Verification items for the finished model (mm, model axes). A direction names the side the tool comes from. Round coordinates to 2 decimals unless told otherwise and drop trailing zeros. Loops run counter-clockwise (first coordinate to the right, second up) from the corner with the lowest first, then second, coordinate; pieces in that order, holes last. Notation, with made-up numbers: (84, -32.75) - (138, -32.75) arc R20 cw to (138, -6.75) - close; hole circle Ø3 at (29.25, -35). An arc over 180 degrees is marked (long way). Use CSV: the item, a comma, the result in double quotes.
```python
from build123d import *

# Parameters (mm, degrees)
F0_W          = 105.625689
F0_H          = 88.043314
F0_R          = 1.5
F1_DEPTH      = 35
F0_W_2        = 44.878527
F2_DEPTH      = 26
F3_SIZE       = 5
F4_W          = 102.581762
F4_H          = 82.043314
F4_W_2        = 41.922454
F5_DEPTH      = 25
F6_R          = 5
F7_W          = 50
F7_H          = 14
F8_DEPTH      = 3
F9_DEPTH      = 25
F9_DEPTH_BACK = 3
F10_W         = 88.043314
F10_H         = 21
F11_DEPTH     = 25


with BuildPart() as f1:
    # F0 (on Top) → F1 (new body)
    with BuildSketch(Plane.XY):
        with Locations((-22.055275, 0)):
            Rectangle(F0_W, F0_H)
        with Locations((-20, -35.20183)):
            Circle(F0_R, mode=Mode.SUBTRACT)
        with Locations((0, -35.20183)):
            Circle(F0_R, mode=Mode.SUBTRACT)
        with Locations((20, -35.20183)):
            Circle(F0_R, mode=Mode.SUBTRACT)
        with Locations((-20, 35.20183)):
            Circle(F0_R, mode=Mode.SUBTRACT)
        with Locations((0, 35.20183)):
            Circle(F0_R, mode=Mode.SUBTRACT)
        with Locations((20, 35.20183)):
            Circle(F0_R, mode=Mode.SUBTRACT)
        with Locations((-20, 35.20183)):
            Circle(F0_R)
        with Locations((0, 35.20183)):
            Circle(F0_R)
        with Locations((20, 35.20183)):
            Circle(F0_R)
        with Locations((20, -35.20183)):
            Circle(F0_R)
        with Locations((0, -35.20183)):
            Circle(F0_R)
        with Locations((-20, -35.20183)):
            Circle(F0_R)
    extrude(amount=F1_DEPTH)

    # F0 (on Top) → F2 (join)
    with BuildSketch(Plane.XY):
        with Locations((53.196832, 0)):
            Rectangle(F0_W_2, F0_H)
    extrude(amount=F2_DEPTH)

    # F3
    f3_edges = [f1.edges().sort_by_distance(p)[0] for p in [
        (30.757569, 0, 35),
    ]]
    chamfer(f3_edges, length=F3_SIZE)

    # F4 (on Top) → F5 (cut)
    with BuildSketch(Plane.XY):
        with Locations((-20.577239, 0)):
            Rectangle(F4_W, F4_H)
        with Locations((51.674869, 0)):
            Rectangle(F4_W_2, F4_H)
    extrude(amount=F5_DEPTH, mode=Mode.SUBTRACT)

    # F6
    f6_edges = [f1.edges().sort_by_distance(p)[0] for p in [
        (53.196833, -44.021657, 26),
        (75.636096, 0, 26),
        (53.196833, 44.021657, 26),
    ]]
    fillet(f6_edges, radius=F6_R)

    # F7 (on face) → F8 (cut)
    with BuildSketch(Plane(origin=(-74.86812, 0, 0), x_dir=(0, -1, 0), z_dir=(-1, 0, 0))):
        with Locations((-5.428568, 10)):
            Rectangle(F7_W, F7_H)
    extrude(amount=-F8_DEPTH, mode=Mode.SUBTRACT)

    # F0 (on Top) → F9 (join, two sides)
    with BuildSketch(Plane.XY) as f9_sk:
        with Locations((-20, -35.20183)):
            Circle(F0_R)
        with Locations((0, -35.20183)):
            Circle(F0_R)
        with Locations((20, -35.20183)):
            Circle(F0_R)
        with Locations((-20, 35.20183)):
            Circle(F0_R)
        with Locations((20, 35.20183)):
            Circle(F0_R)
        with Locations((0, 35.20183)):
            Circle(F0_R)
    extrude(amount=F9_DEPTH)
    extrude(f9_sk.sketch, amount=-F9_DEPTH_BACK)

    # F10 (on face) → F11 (cut)
    with BuildSketch(Plane.YZ.offset(75.636096)):
        with Locations((0, 10.5)):
            Rectangle(F10_W, F10_H)
    extrude(amount=-F11_DEPTH, mode=Mode.SUBTRACT)


solid = f1.part
```
1) Gauge pin test, flat ends, axial feed: pin 1 Ø1.5 at (x, y) = (-5, 27.5) entering from -Z; pin 2 Ø20 at (y, z) = (-3.5, 7.5) entering from +X; pin 3 Ø3.5 at (x, y) = (-73, 12.5) entering from -Z. Record the tip position at first contact, or that the pin passes through.
Returned:
pin 1,"stops at z = 25"
pin 2,"stops at x = -71.87"
pin 3,"stops at z = 0"
2) Cross-section at D-D, the plane y = -32. Record the cut outline in (x, z), then the cut area to 3 significant figures.
Returned:
outline,"(-74.87, 0) - (-71.87, 0) - (-71.87, 25) - (72.64, 25) - (72.64, 21) - (75.64, 21) arc R5 ccw to (70.64, 26) - (30.76, 26) - (30.76, 30) - (25.76, 35) - (-74.87, 35) - close"
area,"1,170 mm²"
3) Mould release check, pull along Y, two halves, no side actions. Record for faces 5 (the face through (53.51, 42.52, 24.57)), 6 (the face through (-73, 6, 17)), 7 (the face through (53.511, -42.596, 24.496)), 8 (the face through (0, 35, -3)): +Y half, -Y half, draft (parallel to the pull), parting line (faces both ways), or undercut.
Returned:
face 5,"+Y half"
face 6,"undercut"
face 7,"-Y half"
face 8,"draft"
4) Cross-section at B-B, the plane z = 13. Record the cut outline in (x, y).
Returned:
outline,"(-74.87, -44.02) - (50.64, -44.02) - (50.64, -41.02) - (-71.87, -41.02) - (-71.87, -19.57) - (-74.87, -19.57) - close; (-74.87, 30.43) - (-71.87, 30.43) - (-71.87, 41.02) - (50.64, 41.02) - (50.64, 44.02) - (-74.87, 44.02) - close; circle Ø3 at (-20, -35.2); circle Ø3 at (-20, 35.2); circle Ø3 at (0, -35.2); circle Ø3 at (0, 35.2); circle Ø3 at (20, -35.2); circle Ø3 at (20, 35.2)"
5) Access from +Z, -Z, +X, -X, +Y, -Y to the whole of each face (thin tool, end or side, straight path). Record for faces 1 (the face through (50.636, 43, 11)), 2 (the face through (-20, 35, -3)), 3 (the face through (50, 1, 26)), 4 (the face through (-71.868, -1, 18)).
Returned:
face 1,"-Z, +X, +Y, -Y"
face 2,"-Z, +X, -X, +Y, -Y"
face 3,"+Z, +X, +Y, -Y"
face 4,"-Z"
6) Cross-section at C-C, the plane x = -15. Record the cut outline in (y, z).
Returned:
outline,"(-44.02, 0) - (-41.02, 0) - (-41.02, 25) - (41.02, 25) - (41.02, 0) - (44.02, 0) - (44.02, 35) - (-44.02, 35) - close"
7) Thickness scan on probe 1 along X at (y, z) = (-35.5, 10); probe 2 along Y at (x, z) = (38.5, 19.5); probe 3 along Z at (x, y) = (-36, -8). Record the ranges inside material, lowest first. Write a range as [from, to].
Returned:
probe 1,"x = [-74.87, -71.87], [-21.47, -18.53], [-1.47, 1.47], [18.53, 21.47]"
probe 2,"y = [-44.02, -41.02], [41.02, 44.02]"
probe 3,"z = [25, 35]"
8) Cross-section at A-A, the plane y = 18. Record the cut outline in (x, z).
Returned:
outline,"(-74.87, 0) - (-71.87, 0) - (-71.87, 3) - (-74.87, 3) - close; (-74.87, 17) - (-71.87, 17) - (-71.87, 25) - (72.64, 25) - (72.64, 21) - (75.64, 21) arc R5 ccw to (70.64, 26) - (30.76, 26) - (30.76, 30) - (25.76, 35) - (-74.87, 35) - close"
